from build123d import *

# Parameters (mm, degrees)
F0_R     = 16.5
F1_DEPTH = 8
F2_R     = 1.05
F3_DEPTH = 2.5
F4_R     = 1
F5_DEPTH = 2.5
F6_W     = 3
F6_H     = 3
F7_DEPTH = 8.001


with BuildPart() as f1:
    # F0 (on Top) → F1 (new body)
    with BuildSketch(Plane.XY):
        Circle(F0_R)
    extrude(amount=F1_DEPTH)

    # F2 (on face) → F3 (cut)
    with BuildSketch(Plane(origin=(0, 0, 0), x_dir=(1, 0, 0), z_dir=(0, 0, -1))):
        with Locations((0, 15.05)):
            Circle(F2_R)
        with Locations((15, 0.05)):
            Circle(F2_R)
        with Locations((0, -14.95)):
            Circle(F2_R)
    extrude(amount=-F3_DEPTH, mode=Mode.SUBTRACT)

    # F4 (on face) → F5 (join)
    with BuildSketch(Plane.XY.offset(8)):
        with Locations((0, 15)):
            Circle(F4_R)
        with Locations((15, 0)):
            Circle(F4_R)
        with Locations((0, -15)):
            Circle(F4_R)
    extrude(amount=F5_DEPTH)

    # F6 (on face) → F7 (cut, through all)
    with BuildSketch(Plane.XY.offset(8)):
        with Locations((-9.5, 9.5)):
            Rectangle(F6_W, F6_H)
        with Locations((-9.5, 4.75)):
            Rectangle(F6_W, F6_H)
        with Locations((-9.5, 0)):
            Rectangle(F6_W, F6_H)
        with Locations((-9.5, -4.75)):
            Rectangle(F6_W, F6_H)
        with Locations((-9.5, -9.5)):
            Rectangle(F6_W, F6_H)
        with Locations((-4.75, 9.5)):
            Rectangle(F6_W, F6_H)
        with Locations((-4.75, 4.75)):
            Rectangle(F6_W, F6_H)
        with Locations((-4.75, 0)):
            Rectangle(F6_W, F6_H)
        with Locations((-4.75, -4.75)):
            Rectangle(F6_W, F6_H)
        with Locations((-4.75, -9.5)):
            Rectangle(F6_W, F6_H)
        with Locations((0, 9.5)):
            Rectangle(F6_W, F6_H)
        with Locations((0, 4.75)):
            Rectangle(F6_W, F6_H)
        Rectangle(F6_W, F6_H)
        with Locations((0, -4.75)):
            Rectangle(F6_W, F6_H)
        with Locations((0, -9.5)):
            Rectangle(F6_W, F6_H)
        with Locations((4.75, 9.5)):
            Rectangle(F6_W, F6_H)
        with Locations((4.75, 4.75)):
            Rectangle(F6_W, F6_H)
        with Locations((4.75, 0)):
            Rectangle(F6_W, F6_H)
        with Locations((4.75, -4.75)):
            Rectangle(F6_W, F6_H)
        with Locations((4.75, -9.5)):
            Rectangle(F6_W, F6_H)
        with Locations((9.5, 9.5)):
            Rectangle(F6_W, F6_H)
        with Locations((9.5, 4.75)):
            Rectangle(F6_W, F6_H)
        with Locations((9.5, 0)):
            Rectangle(F6_W, F6_H)
        with Locations((9.5, -4.75)):
            Rectangle(F6_W, F6_H)
        with Locations((9.5, -9.5)):
            Rectangle(F6_W, F6_H)
    extrude(amount=-F7_DEPTH, mode=Mode.SUBTRACT)


solid = f1.part
Can you work these out from the model? Positions are in its coordinate system, mm. A direction names the side the tool comes from. Round coordinates to 2 decimals unless told otherwise and drop trailing zeros. Loops run counter-clockwise (first coordinate to the right, second up) from the corner with the lowest first, then second, coordinate; pieces in that order, holes last. Notation, with made-up numbers: (80, 68) - (130, 68) arc R25 ccw to (130, 90) - close; hole circle Ø6 at (44, 9.5). An arc over 180 degrees is marked (long way). Write item = value, one per line. Start each with the question number.
(1) If we section it at B-B (y = 4.5): Please give me the cut outline in (x, z).
(2) If I drill on probe 1 along X at (y, z) = (-4, 2); probe 2 along Y at (x, z) = (-9, 6.5); probe 3 along Y at (x, z) = (-9.5, 3.25), over which ranges is the centre line in solid material (lowest first)? Write a range as [from, to].
(3) If we section it at D-D (z = 1.5): Give the number of separate pieces and of enclosed holes in the cut face, and give its area (3 significant figures).
(4) If we section it at A-A (x = 10): Please give me the cut outline in (y, z).
(5) For P1, Ø3.5, axis at y = 5, z = 4, coming from the -X side; P2, Ø1.5, axis at y = 10.5, z = 2.5, coming from the -X side; P3, Ø2.5, axis at x = 4, z = 3, coming from the -Y side, each with a flat end and sliding along its axis, tell me the tip position at first contact or that it passes through.
(6) If we section it at C-C (z = 9.75): Please give me the cut outline in (x, y), and give its area (3 significant figures).
(7) For faces 1 (the face through (0, -14, 1)), 2 (the face through (-5, 11, 4)), which set-ups out of +Z, -Z, +X, -X, +Y, -Y let a thin tool reach every point of the face, with its end or its side?
Ans:
q1.outline = (-15.87, 0) - (-11, 0) - (-11, 8) - (-15.87, 8) - close; (-8, 0) - (-6.25, 0) - (-6.25, 8) - (-8, 8) - close; (-3.25, 0) - (-1.5, 0) - (-1.5, 8) - (-3.25, 8) - close; (1.5, 0) - (3.25, 0) - (3.25, 8) - (1.5, 8) - close; (6.25, 0) - (8, 0) - (8, 8) - (6.25, 8) - close; (11, 0) - (15.87, 0) - (15.87, 8) - (11, 8) - close
q2.probe_1 = [-16.01, -11], [-8, -6.25], [-3.25, -1.5], [1.5, 3.25], [6.25, 8], [11, 16.01]
q2.probe_2 = [-13.83, -11], [-8, -6.25], [-3.25, -1.5], [1.5, 3.25], [6.25, 8], [11, 13.83]
q2.probe_3 = [-13.49, -11], [-8, -6.25], [-3.25, -1.5], [1.5, 3.25], [6.25, 8], [11, 13.49]
q3.separate_pieces = 1
q3.enclosed_holes = 28
q3.area = 620 mm²
q4.outline = (-13.12, 0) - (-11, 0) - (-11, 8) - (-13.12, 8) - close; (-8, 0) - (-6.25, 0) - (-6.25, 8) - (-8, 8) - close; (-3.25, 0) - (-1.5, 0) - (-1.5, 8) - (-3.25, 8) - close; (1.5, 0) - (3.25, 0) - (3.25, 8) - (1.5, 8) - close; (6.25, 0) - (8, 0) - (8, 8) - (6.25, 8) - close; (11, 0) - (13.12, 0) - (13.12, 8) - (11, 8) - close
q5.P1 = -16.18
q5.P2 = -13.31
q5.P3 = -16.27
q6.outline = circle Ø2 at (0, -15); circle Ø2 at (0, 15); circle Ø2 at (15, 0)
q6.area = 9.42 mm²
q7.face_1 = -Z
q7.face_2 = +Z, -Z
